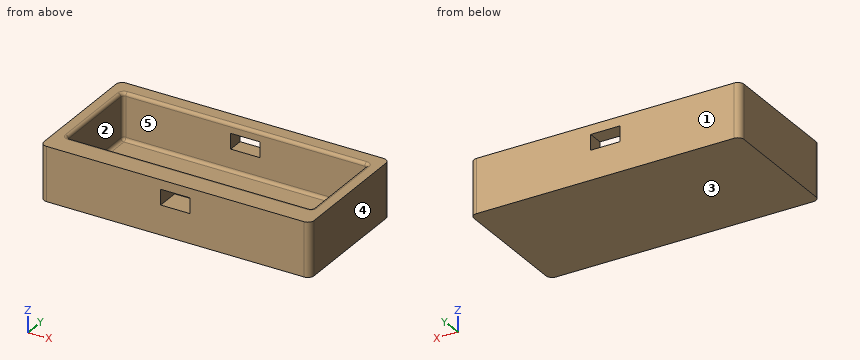
from build123d import *

# Parameters (mm, degrees)
F0_W     = 100.965
F0_H     = 38.1
F1_DEPTH = 19.05
F2_W     = 50.4825
F2_H     = 20.6375
F2_H_2   = 17.4625
F3_DEPTH = 3.175
F4_W     = 12.065
F4_H     = 6.35
F5_DEPTH = 53.976
F6_R     = 1.27


with BuildPart() as f1:
    # F0 (on Top) → F1 (new body)
    with BuildSketch(Plane.XY):
        with BuildLine():
            ThreePointArc((0, 2.54), (0.7439487758, 0.7439487758), (2.54, 0))
            Line((2.54, 0), (108.585, 0))
            ThreePointArc((108.585, 0), (110.3810512242, 0.7439487758), (111.125, 2.54))
            Line((111.125, 2.54), (111.125, 51.435))
            ThreePointArc((111.125, 51.435), (110.3810512242, 53.2310512242), (108.585, 53.975))
            Line((108.585, 53.975), (2.54, 53.975))
            ThreePointArc((2.54, 53.975), (0.7439487758, 53.2310512242), (0, 51.435))
            Line((0, 51.435), (0, 2.54))
        make_face()
        with Locations((55.5625, 28.575)):
            Rectangle(F0_W, F0_H, mode=Mode.SUBTRACT)
    extrude(amount=-F1_DEPTH)

    # F2 (on face) → F3 (join)
    with BuildSketch(Plane(origin=(0, 0, -19.05), x_dir=(1, 0, 0), z_dir=(0, 0, -1))):
        with BuildLine():
            ThreePointArc((0, -51.435), (0.7439487758, -53.2310512242), (2.54, -53.975))
            Line((2.54, -53.975), (55.5625, -53.975))
            Line((55.5625, -53.975), (55.5625, -47.625))
            Line((55.5625, -47.625), (5.08, -47.625))
            Line((5.08, -47.625), (5.08, -26.9875))
            Line((5.08, -26.9875), (0, -26.9875))
            Line((0, -26.9875), (0, -51.435))
        make_face()
        with BuildLine():
            Line((55.5625, -47.625), (55.5625, -53.975))
            Line((55.5625, -53.975), (108.585, -53.975))
            ThreePointArc((108.585, -53.975), (110.3810512242, -53.2310512242), (111.125, -51.435))
            Line((111.125, -51.435), (111.125, -26.9875))
            Line((111.125, -26.9875), (106.045, -26.9875))
            Line((106.045, -26.9875), (106.045, -47.625))
            Line((106.045, -47.625), (55.5625, -47.625))
        make_face()
        with BuildLine():
            Line((0, -2.54), (0, -26.9875))
            Line((0, -26.9875), (5.08, -26.9875))
            Line((5.08, -26.9875), (5.08, -9.525))
            Line((5.08, -9.525), (55.5625, -9.525))
            Line((55.5625, -9.525), (55.5625, 0))
            Line((55.5625, 0), (2.54, 0))
            ThreePointArc((2.54, 0), (0.7439487758, -0.7439487758), (0, -2.54))
        make_face()
        with BuildLine():
            Line((106.045, -26.9875), (111.125, -26.9875))
            Line((111.125, -26.9875), (111.125, -2.54))
            ThreePointArc((111.125, -2.54), (110.3810512242, -0.7439487758), (108.585, 0))
            Line((108.585, 0), (55.5625, 0))
            Line((55.5625, 0), (55.5625, -9.525))
            Line((55.5625, -9.525), (106.045, -9.525))
            Line((106.045, -9.525), (106.045, -26.9875))
        make_face()
        with Locations((30.32125, -37.30625)):
            Rectangle(F2_W, F2_H)
        with Locations((30.32125, -18.25625)):
            Rectangle(F2_W, F2_H_2)
        with Locations((80.80375, -18.25625)):
            Rectangle(F2_W, F2_H_2)
        with Locations((80.80375, -37.30625)):
            Rectangle(F2_W, F2_H)
    extrude(amount=F3_DEPTH)

    # F4 (on face) → F5 (cut, through all)
    with BuildSketch(Plane(origin=(0, 53.975, 0), x_dir=(-1, 0, 0), z_dir=(0, 1, 0))):
        with Locations((-55.5625, -6.985)):
            Rectangle(F4_W, F4_H)
    extrude(amount=-F5_DEPTH, mode=Mode.SUBTRACT)

    # F6
    f6_edges = [f1.edges().sort_by_distance(p)[0] for p in [
        (5.08, 47.625, -9.525),
        (106.045, 47.625, -9.525),
        (5.08, 9.525, -9.525),
        (106.045, 9.525, -9.525),
        (55.5625, 9.525, -19.05),
        (106.045, 28.575, -19.05),
        (55.5625, 47.625, -19.05),
        (5.08, 28.575, -19.05),
        (106.045, 28.575, 0),
        (5.08, 28.575, 0),
        (55.5625, 47.625, 0),
        (55.5625, 9.525, 0),
    ]]
    fillet(f6_edges, radius=F6_R)


solid = f1.part
The listing builds one solid part. Answer for the finished solid, in the listing's coordinates (mm). Face numbers are marked on the shaded views. A direction names the side the tool comes from. Round coordinates to 2 decimals unless told otherwise and drop trailing zeros. Order: outer loops, then holes, each group sorted by start corner. A loop starts at its lowest first (then second) coordinate and runs counter-clockwise, first axis right, second up. Notation, with made-up numbers: (79.5, -6.75) - (126.5, -6.75) arc R27 ccw to (126.5, 26.25) - close; hole circle Ø11 at (67.25, -36.75). An arc over 180 degrees is marked (long way). Write item = value, one per line. Start each with the question number.
1) Straight lines are drawn through the part: L1, parallel to Y at x = 64, z = -5.5 (3 decimals); L2, parallel to X at y = 27, z = -13.5 (3 decimals); L3, parallel to Z at x = 50, y = 4.5 (3 decimals). For each, find the intervals that lie inside material, in ascending order.
2) Section C-C, the plane x = 30 is taken. Write down the section's boundary in (y, z) (3 decimals), plus the area to 3 significant figures.
3) Given pin 1 (8 mm diameter, centred on x = 44, y = 7, fed in from +Z), flat-ended and moving along its own axis, determine where the tip first touches the part or whether it passes through.
4) For the marked faces 4 and 5, determine the directions among +Z, -Z, +X, -X, +Y, -Y from which every point of the face is accessible in a straight line to the end or side of a thin tool.
5) Section B-B, the plane y = 4 is taken. Write down the section's boundary in (x, z) (3 decimals).
6) For a pull along Y with two mould halves and no side action, classify the marked faces 1, 2 and 3 as released by +Y, released by -Y, zero draft, split by the parting line, or undercut.
7) Section A-A, the plane z = -12.5 is taken. Write down the section's boundary in (x, y) (3 decimals), plus the area to 3 significant figures.
8) Section D-D, the plane y = 40.5 is taken. Write down the section's boundary in (x, z) (3 decimals), plus the area to 3 significant figures.
Results list:
q1.L1 = 0 to 9.525, 47.625 to 53.975
q1.L2 = 0 to 5.08, 106.045 to 111.125
q1.L3 = -22.225 to -10.16, -3.81 to 0
q2.outline = (0, -22.225) - (53.975, -22.225) - (53.975, 0) - (48.895, 0) arc R1.27 ccw to (47.625, -1.27) - (47.625, -17.78) arc R1.27 cw to (46.355, -19.05) - (10.795, -19.05) arc R1.27 cw to (9.525, -17.78) - (9.525, -1.27) arc R1.27 ccw to (8.255, 0) - (0, 0) - close
q2.area = 474 mm^2
q3.pin_1 = 0
q4.face_4 = +Z, -Z, +X, +Y, -Y
q4.face_5 = +Z
q5.outline = (0, -22.225) - (111.125, -22.225) - (111.125, 0) - (0, 0) - close; hole (49.53, -10.16) - (61.595, -10.16) - (61.595, -3.81) - (49.53, -3.81) - close
q6.face_1 = released by +Y
q6.face_2 = undercut
q6.face_3 = zero draft
q7.outline = (0, 2.54) arc R2.54 ccw to (2.54, 0) - (108.585, 0) arc R2.54 ccw to (111.125, 2.54) - (111.125, 51.435) arc R2.54 ccw to (108.585, 53.975) - (2.54, 53.975) arc R2.54 ccw to (0, 51.435) - close; hole (5.08, 10.795) arc R1.27 ccw to (6.35, 9.525) - (104.775, 9.525) arc R1.27 ccw to (106.045, 10.795) - (106.045, 46.355) arc R1.27 ccw to (104.775, 47.625) - (6.35, 47.625) arc R1.27 ccw to (5.08, 46.355) - close
q7.area = 2,150 mm^2
q8.outline = (0, -22.225) - (111.125, -22.225) - (111.125, 0) - (107.315, 0) arc R1.27 ccw to (106.045, -1.27) - (106.045, -17.78) arc R1.27 cw to (104.775, -19.05) - (6.35, -19.05) arc R1.27 cw to (5.08, -17.78) - (5.08, -1.27) arc R1.27 ccw to (3.81, 0) - (0, 0) - close
q8.area = 546 mm^2
